Autodesk Inventor part; units mm, degrees
ref_plane "YZ Plane" through (0, 0, 0) normal (1, 0, 0) x (0, 1, 0)
ref_plane "XZ Plane" through (0, 0, 0) normal (0, 1, 0) x (-1, 0, 0)
ref_plane "XY Plane" through (0, 0, 0) normal (0, 0, 1) x (1, 0, 0)
sketch "Sketch_1" plane through (0, 0, 0) normal (0, 0, 1) x (1, 0, 0)
  arc A0 (-12.7, -10.5664) -> (-10.5664, -12.7) centre (-10.592, -10.592) ccw
  arc A1 (-9.5504, -12.7) -> (-10.5664, -12.7) centre (-10.0584, -12.7) ccw
  line L0 (-9.5504, -12.7) -> (-6.3246, -12.7)
  arc A2 (-5.3086, -12.7) -> (-6.3246, -12.7) centre (-5.8166, -12.7) ccw
  line L1 (-5.3086, -12.7) -> (-4.3023, -12.7)
  arc A3 (-4.3023, -12.7) -> (-4.3023, -10.4902) centre (-4.3023, -11.5951) ccw
  line L2 (-4.3023, -10.4902) -> (-6.4748, -10.4902)
  arc A4 (-7.1932, -8.7558) -> (-6.4748, -10.4902) centre (-6.4748, -9.4742) ccw
  line L3 (-7.1932, -8.7558) -> (-3.8759, -5.4384)
  arc A5 (-1.6308, -4.5085) -> (-3.8759, -5.4384) centre (-1.6308, -7.6835) ccw
  line L4 (-1.6308, -4.5085) -> (1.6308, -4.5085)
  arc A6 (3.8759, -5.4384) -> (1.6308, -4.5085) centre (1.6308, -7.6835) ccw
  line L5 (3.8759, -5.4384) -> (7.1932, -8.7558)
  arc A7 (6.4748, -10.4902) -> (7.1932, -8.7558) centre (6.4748, -9.4742) ccw
  line L6 (6.4748, -10.4902) -> (4.3023, -10.4902)
  arc A8 (4.3023, -10.4902) -> (4.3023, -12.7) centre (4.3023, -11.5951) ccw
  line L7 (4.3023, -12.7) -> (5.3086, -12.7)
  arc A9 (6.3246, -12.7) -> (5.3086, -12.7) centre (5.8166, -12.7) ccw
  line L8 (6.3246, -12.7) -> (9.5504, -12.7)
  arc A10 (10.5664, -12.7) -> (9.5504, -12.7) centre (10.0584, -12.7) ccw
  arc A11 (10.5664, -12.7) -> (12.7, -10.5664) centre (10.592, -10.592) ccw
  arc A12 (12.7, -9.5504) -> (12.7, -10.5664) centre (12.7, -10.0584) ccw
  line L9 (12.7, -9.5504) -> (12.7, -6.3246)
  arc A13 (12.7, -5.3086) -> (12.7, -6.3246) centre (12.7, -5.8166) ccw
  line L10 (12.7, -5.3086) -> (12.7, -4.3023)
  arc A14 (12.7, -4.3023) -> (10.4902, -4.3023) centre (11.5951, -4.3023) ccw
  line L11 (10.4902, -4.3023) -> (10.4902, -6.4748)
  arc A15 (8.7558, -7.1932) -> (10.4902, -6.4748) centre (9.4742, -6.4748) ccw
  line L12 (8.7558, -7.1932) -> (5.4384, -3.8759)
  arc A16 (4.5085, -1.6308) -> (5.4384, -3.8759) centre (7.6835, -1.6308) ccw
  line L13 (4.5085, -1.6308) -> (4.5085, 1.6308)
  arc A17 (5.4384, 3.8759) -> (4.5085, 1.6308) centre (7.6835, 1.6308) ccw
  line L14 (5.4384, 3.8759) -> (8.7558, 7.1932)
  arc A18 (10.4902, 6.4748) -> (8.7558, 7.1932) centre (9.4742, 6.4748) ccw
  line L15 (10.4902, 6.4748) -> (10.4902, 4.3023)
  arc A19 (10.4902, 4.3023) -> (12.7, 4.3023) centre (11.5951, 4.3023) ccw
  line L16 (12.7, 4.3023) -> (12.7, 5.3086)
  arc A20 (12.7, 6.3246) -> (12.7, 5.3086) centre (12.7, 5.8166) ccw
  line L17 (12.7, 6.3246) -> (12.7, 9.5504)
  arc A21 (12.7, 10.5664) -> (12.7, 9.5504) centre (12.7, 10.0584) ccw
  arc A22 (12.7, 10.5664) -> (10.5664, 12.7) centre (10.592, 10.592) ccw
  arc A23 (9.5504, 12.7) -> (10.5664, 12.7) centre (10.0584, 12.7) ccw
  line L18 (9.5504, 12.7) -> (6.3246, 12.7)
  arc A24 (5.3086, 12.7) -> (6.3246, 12.7) centre (5.8166, 12.7) ccw
  line L19 (5.3086, 12.7) -> (4.3023, 12.7)
  arc A25 (4.3023, 12.7) -> (4.3023, 10.4902) centre (4.3023, 11.5951) ccw
  line L20 (4.3023, 10.4902) -> (6.4748, 10.4902)
  arc A26 (7.1932, 8.7558) -> (6.4748, 10.4902) centre (6.4748, 9.4742) ccw
  line L21 (7.1932, 8.7558) -> (3.8759, 5.4384)
  arc A27 (1.6308, 4.5085) -> (3.8759, 5.4384) centre (1.6308, 7.6835) ccw
  line L22 (1.6308, 4.5085) -> (-1.6308, 4.5085)
  arc A28 (-3.8759, 5.4384) -> (-1.6308, 4.5085) centre (-1.6308, 7.6835) ccw
  line L23 (-3.8759, 5.4384) -> (-7.1932, 8.7558)
  arc A29 (-6.4748, 10.4902) -> (-7.1932, 8.7558) centre (-6.4748, 9.4742) ccw
  line L24 (-6.4748, 10.4902) -> (-4.3023, 10.4902)
  arc A30 (-4.3023, 10.4902) -> (-4.3023, 12.7) centre (-4.3023, 11.5951) ccw
  line L25 (-4.3023, 12.7) -> (-5.3086, 12.7)
  arc A31 (-6.3246, 12.7) -> (-5.3086, 12.7) centre (-5.8166, 12.7) ccw
  line L26 (-6.3246, 12.7) -> (-9.5504, 12.7)
  arc A32 (-10.5664, 12.7) -> (-9.5504, 12.7) centre (-10.0584, 12.7) ccw
  arc A33 (-10.5664, 12.7) -> (-12.7, 10.5664) centre (-10.592, 10.592) ccw
  arc A34 (-12.7, 9.5504) -> (-12.7, 10.5664) centre (-12.7, 10.0584) ccw
  line L27 (-12.7, 9.5504) -> (-12.7, 6.3246)
  arc A35 (-12.7, 5.3086) -> (-12.7, 6.3246) centre (-12.7, 5.8166) ccw
  line L28 (-12.7, 5.3086) -> (-12.7, -5.3086)
  arc A36 (-12.7, -6.3246) -> (-12.7, -5.3086) centre (-12.7, -5.8166) ccw
  line L29 (-12.7, -6.3246) -> (-12.7, -9.5504)
  arc A37 (-12.7, -10.5664) -> (-12.7, -9.5504) centre (-12.7, -10.0584) ccw
  circle A38 centre (0, 0) radius 2.6035
  arc A39 (-10.4902, -6.4135) -> (-9.4742, -7.4295) centre (-9.4742, -6.4135) ccw
  arc A40 (-9.4742, -7.4295) -> (-8.6945, -7.1319) centre (-9.4638, -6.2865) ccw
  line L30 (-8.6945, -7.1319) -> (-5.4384, -3.8759)
  arc A41 (-5.4384, -3.8759) -> (-4.5085, -1.6308) centre (-7.6835, -1.6308) ccw
  line L31 (-4.5085, -1.6308) -> (-4.5085, 1.6308)
  arc A42 (-4.5085, 1.6308) -> (-5.4384, 3.8759) centre (-7.6835, 1.6308) ccw
  line L32 (-5.4384, 3.8759) -> (-8.6945, 7.1319)
  arc A43 (-8.6945, 7.1319) -> (-9.4742, 7.4295) centre (-9.4638, 6.2865) ccw
  arc A44 (-9.4742, 7.4295) -> (-10.4902, 6.4135) centre (-9.4742, 6.4135) ccw
  line L33 (-10.4902, 6.4135) -> (-10.4902, -6.4135)
extrude "Extrusion1" add sketch "Sketch_1" against normal blind 1219.2
properties part number "1003-48-CL"
The model under review builds one solid part; all positions refer to its coordinate system, in mm. Round coordinates to 2 decimals unless told otherwise and drop trailing zeros.
1) Consider section A-A on z = -696.5. Give the number of separate pieces and of enclosed holes in the cut face, then the cut area to 3 significant figures.
Values follow:
separate pieces: 1
enclosed holes: 2
area: 296 mm2
2) Clearance check with flat-ended pins moving along their axes: P1, Ø1, axis at y = 0.5, z = -497, coming from the +X side; P2, Ø1.5, axis at x = 5.5, y = -2.5, coming from the +Z side. State where each tip first meets the part, or that it passes through.
Values follow:
P1: stops at x = 4.51
P2: passes through
3) Wall thickness on line 1 along Y through (x, z) = (0, -629); line 2 along X through (y, z) = (11, -885); line 3 along X through (y, z) = (0.5, -727.5): over which ranges is each line inside the solid? List them lowest first.
Values follow:
line 1: y = -4.51 to -2.6, 2.6 to 4.51
line 2: x = -12.66 to -3.37, 3.37 to 12.66
line 3: x = -12.7 to -10.49, -4.51 to -2.56, 2.56 to 4.51
